Build history of the part. All positions in model axes, mm. A direction names the side the tool comes from. Round coordinates to 2 decimals unless told otherwise and drop trailing zeros. Write each loop counter-clockwise with the first axis right and the second up, starting at its lowest first coordinate (ties: lowest second). Pieces come first, ordered by that corner, then holes. Notation, with made-up numbers: M 20.25,-1.5 L 69.25,-1.5 A16 cw 69.25,12.5 Z; hole C -15,65.25 d6. An arc over 180 degrees is marked long. Write item = value, one per line. Start each with the question number.
Q1. Tool access for faces 4 (the flat face through (10.16, 0, 0)), 5 (the conical face through (2.79, -0.03, -5.53)): list every direction of +Z, -Z, +X, -X, +Y, -Y with a clear straight run to the whole face (end or side of a thin tool).
Q2. Band-saw the part on B-B on y = 8.25. Write the cut outline in (x, z), plus the area to 3 significant figures.
Q3. Pull direction Z, two halves, no side cores. Call faces 1 (the cylindrical face through (-6.28, -4.02, -4.38)), 2 (the flat face through (-2, 10.16, -6)), 3 (the flat face through (0, 0, -10.16)): released by +Z, released by -Z, zero draft, split by the parting line, or undercut.
Q4. Band-saw the part on A-A on z = 4.5. State how many separate pieces and enclosed holes the cut face has, plus the area to 3 significant figures.
Q5. Probe L1, parallel to Y at x = -6.75, z = 0; L2, parallel to Z at x = -4, y = -2.5. List the from-to ranges inside material, lowest first.
Q6. Drop flat-ended pins along their axis: P1, Ø3, axis at y = 0, z = 2.5, coming from the -X side; P2, Ø5, axis at x = -1.5, z = -1, coming from the -Y side; P3, Ø2, axis at y = 6.5, z = 7, coming from the -X side. Give the stop position or say it passes through.
```python
from build123d import *

# Parameters (mm, degrees)
R_P_TITION_START                   = -7.62
R_P_TITION_CIRCULAIRE5_OUTLINE_W   = 3.84
R_P_TITION_CIRCULAIRE5_OUTLINE_H   = 18
R_P_TITION_CIRCULAIRE5_DEPTH       = 15.24
R_P_TITION_START_2                 = -12.7
R_P_TITION_CIRCULAIRE5_2_OUTLINE_W = 19.16
R_P_TITION_CIRCULAIRE5_2_OUTLINE_H = 18
R_P_TITION_CIRCULAIRE5_2_DEPTH     = 2.54
R_P_TITION_START_3                 = 10.16
R_P_TITION_CIRCULAIRE5_3_OUTLINE_W = 19.16
R_P_TITION_CIRCULAIRE5_3_OUTLINE_H = 18
R_P_TITION_CIRCULAIRE5_3_DEPTH     = 2.54
R_P_TITION_CIRCULAIRE6_OUTLINE_W   = 18
R_P_TITION_CIRCULAIRE6_OUTLINE_H   = 18
R_P_TITION_CIRCULAIRE6_DEPTH       = 2.54
R_P_TITION_CIRCULAIRE6_2_OUTLINE_W = 18
R_P_TITION_CIRCULAIRE6_2_OUTLINE_H = 18
R_P_TITION_CIRCULAIRE6_2_DEPTH     = 2.54
CONG_1_R                           = 1
R_P_TITION_CIRCULAIRE7_COUNT       = 3
R_P_TITION_CIRCULAIRE7_ANGLE       = 180


# Read off the part's stored shape, not the designer's step: Répétition circulaire5, Répétition circulaire6
with BuildPart() as part:
    # Esquisse1 → Révolution1 (revolve)
    with BuildSketch(Plane.XY):
        with BuildLine():
            Line((0, -12.7), (0, 12.7))
            ThreePointArc((0, 12.7), (12.7, 0), (0, -12.7))
        make_face()
    revolve(axis=Axis((0, -12.7, 0), (0, 1, 0)))

    # Enlèv. mat.-Surface1
    split(bisect_by=Plane(origin=(0, 10.16, 0), x_dir=(1, 0, 0), z_dir=(0, 1, 0)), keep=Keep.BOTTOM)

    # Répétition circulaire5 outline → Répétition circulaire5 (cut)
    with BuildSketch(Plane.YZ.offset(R_P_TITION_START)):
        with Locations((-12.08, 0)):
            Rectangle(R_P_TITION_CIRCULAIRE5_OUTLINE_W, R_P_TITION_CIRCULAIRE5_OUTLINE_H)
    extrude(amount=R_P_TITION_CIRCULAIRE5_DEPTH, mode=Mode.SUBTRACT)

    # R_p_tition circulaire5 2 outline → R_p_tition circulaire5 2 (cut)
    with BuildSketch(Plane.YZ.offset(R_P_TITION_START_2)):
        with Locations((-0.58, 0)):
            Rectangle(R_P_TITION_CIRCULAIRE5_2_OUTLINE_W, R_P_TITION_CIRCULAIRE5_2_OUTLINE_H)
    extrude(amount=R_P_TITION_CIRCULAIRE5_2_DEPTH, mode=Mode.SUBTRACT)

    # R_p_tition circulaire5 3 outline → R_p_tition circulaire5 3 (cut)
    with BuildSketch(Plane.YZ.offset(R_P_TITION_START_3)):
        with Locations((-0.58, 0)):
            Rectangle(R_P_TITION_CIRCULAIRE5_3_OUTLINE_W, R_P_TITION_CIRCULAIRE5_3_OUTLINE_H)
    extrude(amount=R_P_TITION_CIRCULAIRE5_3_DEPTH, mode=Mode.SUBTRACT)

    # Répétition circulaire6 outline → Répétition circulaire6 (cut)
    with BuildSketch(Plane.XY.offset(R_P_TITION_START_2)):
        Rectangle(R_P_TITION_CIRCULAIRE6_OUTLINE_W, R_P_TITION_CIRCULAIRE6_OUTLINE_H)
    extrude(amount=R_P_TITION_CIRCULAIRE6_DEPTH, mode=Mode.SUBTRACT)

    # R_p_tition circulaire6 2 outline → R_p_tition circulaire6 2 (cut)
    with BuildSketch(Plane.XY.offset(R_P_TITION_START_3)):
        Rectangle(R_P_TITION_CIRCULAIRE6_2_OUTLINE_W, R_P_TITION_CIRCULAIRE6_2_OUTLINE_H)
    extrude(amount=R_P_TITION_CIRCULAIRE6_2_DEPTH, mode=Mode.SUBTRACT)

    # Congé1
    cong_1_edges = [part.edges().sort_by_distance(p)[0] for p in [
        (-10.16, 0, -7.62),
        (-7.62, -10.16, 0),
        (10.16, 0, -7.62),
        (0, 7.62, -10.16),
        (0, 7.62, 10.16),
        (-7.62, 10.16, 0),
    ]]
    fillet(cong_1_edges, radius=CONG_1_R)

    # Esquisse2 → Trou taraudé 1/4-18 NPSM1 (revolve, cut)
    with BuildSketch(Plane(origin=(0, 10.16, 0), x_dir=(0, 0, 1), z_dir=(1, 0, 0))):
        Polygon((0, 0), (0, 16.271275175), (5.9436, 12.7), (5.9436, 0), align=None)
    trou_taraud_1_4_18_npsm1 = revolve(axis=Axis((0, 16.51, 0), (0, -1, 0)), mode=Mode.SUBTRACT)

    # Répétition circulaire7: Trou taraudé 1/4-18 NPSM1 ×3 about axis
    r_p_tition_circulaire7_axis = Axis((0, 0, -11.176), (0, 0, 1))
    for i in range(1, R_P_TITION_CIRCULAIRE7_COUNT):
        add(trou_taraud_1_4_18_npsm1.rotate(r_p_tition_circulaire7_axis, i * R_P_TITION_CIRCULAIRE7_ANGLE / (R_P_TITION_CIRCULAIRE7_COUNT - 1)), mode=Mode.SUBTRACT)


solid = part.part
```
Conclusion:
q1.face_4 = +Z, -Z, +X, +Y, -Y
q1.face_5 = -X
q2.outline = C 0,0 d19.31; hole C 0,0 d11.89
q2.area = 182 mm^2
q3.face_1 = undercut
q3.face_2 = zero draft
q3.face_3 = released by -Z
q4.separate_pieces = 3
q4.enclosed_holes = 0
q4.area = 179 mm^2
q5.L1 = -10.16 to -5.94, 5.94 to 10.16
q5.L2 = -10.16 to -5.39, 5.39 to 10.16
q6.P1 = 4.4
q6.P2 = through
q6.P3 = -9.39
